from build123d import *

# Parameters (mm, degrees)
M3_NECK_AND_THREAD_ENVELOPE_SKETCH_R = 1.5
M3_NECK_AND_THREAD_ENVELOPE_DEPTH    = 15.8
ANCHOR_SEATING_COLLAR_SKETCH_R       = 3
ANCHOR_SEATING_COLLAR_DEPTH          = 1
ANCHOR_TAIL_HEX_DRIVE_DEPTH          = 1.6


with BuildPart() as part:
    # M3 neck and thread envelope sketch → M3 neck and thread envelope (new body)
    with BuildSketch(Plane(origin=(0, -90, 0), x_dir=(-1, 0, 0), z_dir=(0, -1, 0))):
        with Locations(Location((23.382685902, 19, 0), (0, 0, 90))):
            Circle(M3_NECK_AND_THREAD_ENVELOPE_SKETCH_R)
    extrude(amount=M3_NECK_AND_THREAD_ENVELOPE_DEPTH)

    # Six millimetre anchor ball profile → Six millimetre anchor ball (revolve)
    with BuildSketch(Plane(origin=(0, -90, 0), x_dir=(-1, 0, 0), z_dir=(0, -1, 0))):
        with BuildLine():
            Line((23.382685902, 16), (23.382685902, 22))
            ThreePointArc((23.382685902, 22), (20.382685902, 19), (23.382685902, 16))
        make_face()
    revolve(axis=Axis((-23.382685902, -90, -29), (0, 0, 1)))

    # Anchor seating collar sketch → Anchor seating collar (add)
    with BuildSketch(Plane(origin=(0, -96.3, 0), x_dir=(-1, 0, 0), z_dir=(0, -1, 0))):
        with Locations(Location((23.382685902, 19, 0), (0, 0, 90))):
            Circle(ANCHOR_SEATING_COLLAR_SKETCH_R)
    extrude(amount=ANCHOR_SEATING_COLLAR_DEPTH)

    # Anchor tail hex drive sketch → Anchor tail hex drive (cut)
    with BuildSketch(Plane(origin=(0, -105.9, 0), x_dir=(1, 0, 0), z_dir=(0, 1, 0))):
        Polygon((-22.516660498, 19), (-22.9496732, 19.75), (-23.815698604, 19.75), (-24.248711306, 19), (-23.815698604, 18.25), (-22.9496732, 18.25), align=None)
    extrude(amount=ANCHOR_TAIL_HEX_DRIVE_DEPTH, mode=Mode.SUBTRACT)


solid = part.part
Could you check a few things on this model? Use its own coordinates, in mm. A direction names the side the tool comes from. Coordinates: 2 decimals unless noted, no trailing zeros. Order: outer loops, then holes, each group sorted by start corner. A loop starts at its lowest first (then second) coordinate and runs counter-clockwise, first axis right, second up.
Q1. Which directions (+Z, -Z, +X, -X, +Y, -Y) give clear straight access to the entire face, cutting with the end or side of a thin tool? Please do faces 1 (the cylindrical face through (-23.3, -96.8, -16)), 2 (the cylindrical face through (-23.32, -101.49, -17.5)), 3 (the flat face through (-22, -96.3, -20)).
Q2. Will this pin go through, and if not, where does the flat tip stop? pin 1 (1 mm diameter, centred on y = -97, z = -20, fed in from +X).
Q3. Suppose I cut it at C-C on y = -100.5. Please give me the cut outline in (x, z), and give its area (3 significant figures).
Q4. Thinking about a two-plate mould opening in Z: for faces 4 (the cylindrical face through (-23.32, -94.42, -17.5)), 5 (the flat face through (-23.4, -105.1, -18.25)), 6 (the flat face through (-23, -104.3, -19)), 7 (the flat face through (-24, -105.8, -20)), which applies, released by +Z, released by -Z, zero draft, split by the parting line, or undercut?
Q5. Please list where these lines run through material, in increasing order: L1, parallel to Y at x = -21.9, z = -20.2; L2, parallel to Y at x = -25.2, z = -20.05; L3, parallel to Z at x = -22.85, y = -102.25.
Q6. Suppose I cut it at B-B on z = -17.95. Please give me the cut outline in (x, y), and give its area (3 significant figures).
Q7. Suppose I cut it at A-A on x = -21.45. Please give me the cut outline in (y, z), and give its area (3 significant figures).
Answer:
1. face 1: +Y, -Y
1. face 2: -Y
1. face 3: none
2. pin 1: stops at x = -20.42
3. outline: circle Ø3 at (-23.38, -19)
3. area: 7.07 mm2
4. face 4: split by the parting line
4. face 5: undercut
4. face 6: undercut
4. face 7: zero draft
5. L1: y = -97.3 to -96.3, -92.32 to -87.68
5. L2: y = -97.3 to -96.3, -92.14 to -87.86
5. L3: z = -20.4 to -17.6
6. outline: (-26.19, -97.3) - (-24.45, -97.3) - (-24.45, -105.8) - (-22.31, -105.8) - (-22.31, -97.3) - (-20.57, -97.3) - (-20.57, -96.3) - (-22.31, -96.3) - (-22.31, -92.6) arc R2.81 ccw (long way) to (-24.45, -92.6) - (-24.45, -96.3) - (-26.19, -96.3) - close
6. area: 56.3 mm2
7. outline: (-97.3, -21.29) - (-96.3, -21.29) - (-96.3, -16.71) - (-97.3, -16.71) - close; circle Ø4.59 at (-90, -19)
7. area: 21.1 mm2
